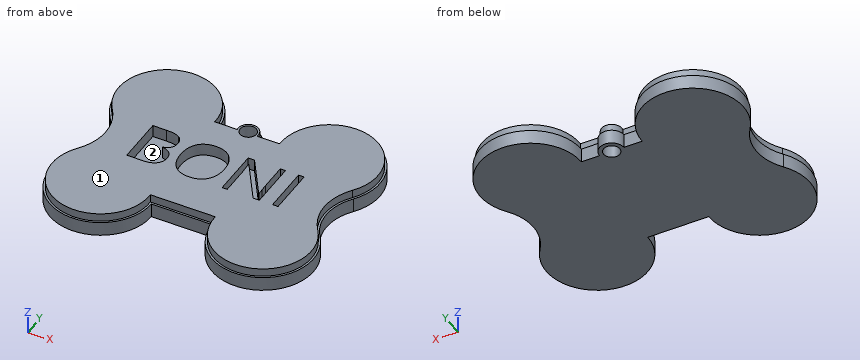
```python
from build123d import *

# Parameters (mm, degrees)
F0_R     = 2
F1_DEPTH = 3.5
F2_R     = 2
F3_DEPTH = 1
F4_W     = 1.3676754668
F4_H     = 11.7681905988
F4_R     = 2
F5_DEPTH = 3


with BuildPart() as f1:
    # F0 (on Top) → F1 (new body)
    with BuildSketch(Plane.XY):
        with BuildLine():
            Line((27, 30), (22.5, 30))
            ThreePointArc((22.5, 30), (6.0471529248, 41.8585412256), (0, 22.5))
            ThreePointArc((0, 22.5), (2.5, 15), (0, 7.5))
            ThreePointArc((0, 7.5), (6.0471529248, -11.8585412256), (22.5, 0))
            Line((22.5, 0), (37.5, 0))
            ThreePointArc((37.5, 0), (53.9528470752, -11.8585412256), (60, 7.5))
            ThreePointArc((60, 7.5), (57.5, 15), (60, 22.5))
            ThreePointArc((60, 22.5), (53.9528470752, 41.8585412256), (37.5, 30))
            Line((37.5, 30), (33, 30))
            ThreePointArc((33, 30), (30, 33), (27, 30))
        make_face()
        with Locations((30, 30)):
            Circle(F0_R, mode=Mode.SUBTRACT)
    extrude(amount=F1_DEPTH)

    # F2 (on face) → F3 (cut)
    with BuildSketch(Plane.XY.offset(3.5)):
        with BuildLine():
            Line((21.9895788083, 0.5), (38.0104211917, 0.5))
            ThreePointArc((38.0104211917, 0.5), (53.5566869022, -11.4608018166), (59.6, 7.2))
            ThreePointArc((59.6, 7.2), (57, 15), (59.6, 22.8))
            ThreePointArc((59.6, 22.8), (53.5566869022, 41.4608018166), (38.0104211917, 29.5))
            Line((38.0104211917, 29.5), (32.4494897428, 29.5))
            ThreePointArc((32.4494897428, 29.5), (30, 32.5), (27.5505102572, 29.5))
            Line((27.5505102572, 29.5), (21.9895788083, 29.5))
            ThreePointArc((21.9895788083, 29.5), (6.4433130978, 41.4608018166), (0.4, 22.8))
            ThreePointArc((0.4, 22.8), (3, 15), (0.4, 7.2))
            ThreePointArc((0.4, 7.2), (6.4433130978, -11.4608018166), (21.9895788083, 0.5))
        make_face()
        with Locations((30, 30)):
            Circle(F2_R, mode=Mode.SUBTRACT)
    extrude(amount=-F3_DEPTH, mode=Mode.SUBTRACT)

    # F4 (on face) → F5 (join)
    with BuildSketch(Plane.XY.offset(2.5)):
        with BuildLine():
            ThreePointArc((0.4, 7.2), (6.4433130978, -11.4608018166), (21.9895788083, 0.5))
            Line((21.9895788083, 0.5), (38.0104211917, 0.5))
            ThreePointArc((38.0104211917, 0.5), (53.5566869022, -11.4608018166), (59.6, 7.2))
            ThreePointArc((59.6, 7.2), (57, 15), (59.6, 22.8))
            ThreePointArc((59.6, 22.8), (53.5566869022, 41.4608018166), (38.0104211917, 29.5))
            Line((38.0104211917, 29.5), (32.4494897428, 29.5))
            ThreePointArc((32.4494897428, 29.5), (30, 32.5), (27.5505102572, 29.5))
            Line((27.5505102572, 29.5), (21.9895788083, 29.5))
            ThreePointArc((21.9895788083, 29.5), (6.4433130978, 41.4608018166), (0.4, 22.8))
            ThreePointArc((0.4, 22.8), (3, 15), (0.4, 7.2))
        make_face()
        with BuildLine():
            Line((10.8878203307, 10.1561439622), (10.8878203307, 21.924334561))
            Line((10.8878203307, 21.924334561), (14.2129974073, 21.924334561))
            add(Edge.make_bspline(
                [(14.2129974073, 21.924334561), (16.554272359, 21.924334561), (17.6012781542, 21.2237550375)],
                knots=[0, 0, 0, 1, 1, 1], degree=2))
            add(Edge.make_bspline(
                [(17.6012781542, 21.2237550375), (18.6482839495, 20.523175514), (18.6482839495, 19.0112630864)],
                knots=[0, 0, 0, 1, 1, 1], degree=2))
            add(Edge.make_bspline(
                [(18.6482839495, 19.0112630864), (18.6482839495, 17.9629694612), (18.0648969566, 17.2829952178)],
                knots=[0, 0, 0, 1, 1, 1], degree=2))
            add(Edge.make_bspline(
                [(18.0648969566, 17.2829952178), (17.4815099636, 16.6030209744), (16.361097858, 16.4021194934)],
                knots=[0, 0, 0, 1, 1, 1], degree=2))
            Line((16.361097858, 16.4021194934), (16.361097858, 16.322274033))
            add(Edge.make_bspline(
                [(16.361097858, 16.322274033), (19.0423599314, 15.8638065507), (19.0423599314, 13.5045019789)],
                knots=[0, 0, 0, 1, 1, 1], degree=2))
            add(Edge.make_bspline(
                [(19.0423599314, 13.5045019789), (19.0423599314, 11.928198051), (17.9760366861, 11.0421710066)],
                knots=[0, 0, 0, 1, 1, 1], degree=2))
            add(Edge.make_bspline(
                [(17.9760366861, 11.0421710066), (16.9097134408, 10.1561439622), (14.9934223912, 10.1561439622)],
                knots=[0, 0, 0, 1, 1, 1], degree=2))
            Line((14.9934223912, 10.1561439622), (10.8878203307, 10.1561439622))
        make_face(mode=Mode.SUBTRACT)
        with BuildLine():
            add(Edge.make_bspline(
                [(30.359810028, 20.4999945739), (31.7841500152, 18.8902070658), (31.7841500152, 16.0569810517)],
                knots=[0, 0, 0, 1, 1, 1], degree=2))
            add(Edge.make_bspline(
                [(31.7841500152, 16.0569810517), (31.7841500152, 13.2314820175), (30.354658708, 11.6126796994)],
                knots=[0, 0, 0, 1, 1, 1], degree=2))
            add(Edge.make_bspline(
                [(30.354658708, 11.6126796994), (28.9251674009, 9.9938773813), (26.3829909681, 9.9938773813)],
                knots=[0, 0, 0, 1, 1, 1], degree=2))
            add(Edge.make_bspline(
                [(26.3829909681, 9.9938773813), (23.7841500152, 9.9938773813), (22.3714004981, 11.5843474393)],
                knots=[0, 0, 0, 1, 1, 1], degree=2))
            add(Edge.make_bspline(
                [(22.3714004981, 11.5843474393), (20.958650981, 13.1748174973), (20.958650981, 16.0724350117)],
                knots=[0, 0, 0, 1, 1, 1], degree=2))
            add(Edge.make_bspline(
                [(20.958650981, 16.0724350117), (20.958650981, 18.9468715861), (22.3752639881, 20.528326834)],
                knots=[0, 0, 0, 1, 1, 1], degree=2))
            add(Edge.make_bspline(
                [(22.3752639881, 20.528326834), (23.7918769952, 22.1097820819), (26.3984449282, 22.1097820819)],
                knots=[0, 0, 0, 1, 1, 1], degree=2))
            add(Edge.make_bspline(
                [(26.3984449282, 22.1097820819), (28.9354700409, 22.1097820819), (30.359810028, 20.4999945739)],
                knots=[0, 0, 0, 1, 1, 1], degree=2))
        make_face(mode=Mode.SUBTRACT)
        with BuildLine():
            Line((43.5987024942, 21.924334561), (43.5987024942, 10.1561439622))
            Line((43.5987024942, 10.1561439622), (42.0378525264, 10.1561439622))
            Line((42.0378525264, 10.1561439622), (35.6064294743, 20.0312244515))
            Line((35.6064294743, 20.0312244515), (35.5420379739, 20.0312244515))
            add(Edge.make_bspline(
                [(35.5420379739, 20.0312244515), (35.6708209746, 18.2926539428), (35.6708209746, 16.8451330156)],
                knots=[0, 0, 0, 1, 1, 1], degree=2))
            Line((35.6708209746, 16.8451330156), (35.6708209746, 10.1561439622))
            Line((35.6708209746, 10.1561439622), (34.4061719083, 10.1561439622))
            Line((34.4061719083, 10.1561439622), (34.4061719083, 21.924334561))
            Line((34.4061719083, 21.924334561), (35.951567916, 21.924334561))
            Line((35.951567916, 21.924334561), (42.3675370081, 12.0878889718))
            Line((42.3675370081, 12.0878889718), (42.4319285084, 12.0878889718))
            add(Edge.make_bspline(
                [(42.4319285084, 12.0878889718), (42.4164745483, 12.3042444129), (42.359810028, 13.4838966988)],
                knots=[0, 0, 0, 1, 1, 1], degree=2))
            add(Edge.make_bspline(
                [(42.359810028, 13.4838966988), (42.3031455078, 14.6635489847), (42.3185994678, 15.1709540072)],
                knots=[0, 0, 0, 1, 1, 1], degree=2))
            Line((42.3185994678, 15.1709540072), (42.3185994678, 21.924334561))
            Line((42.3185994678, 21.924334561), (43.5987024942, 21.924334561))
        make_face(mode=Mode.SUBTRACT)
        with Locations((47.5175692038, 16.0402392616)):
            Rectangle(F4_W, F4_H, mode=Mode.SUBTRACT)
        with Locations((30, 30)):
            Circle(F4_R, mode=Mode.SUBTRACT)
    extrude(amount=F5_DEPTH)


solid = f1.part
```
CAD build for the part. Positions are in the model's coordinates, mm. Face numbers are marked on the shaded views. Coordinates: 2 decimals unless noted, no trailing zeros. Order: outer loops, then holes, each group sorted by start corner. A loop starts at its lowest first (then second) coordinate and runs counter-clockwise, first axis right, second up.
(1) Saw through at C-C, the plane x = 53.5. Write the cut outline in (y, z), and give its area (3 significant figures).
Solution:
outline: (-12, 0) - (42, 0) - (42, 3.5) - (41.48, 3.5) - (41.48, 5.5) - (-11.48, 5.5) - (-11.48, 3.5) - (-12, 3.5) - close
area: 295 mm2
(2) Pin check, flat tips, straight feed: pin 1 Ø1.6 at (x, z) = (24, 4.5) entering from +Y; pin 2 Ø0.9 at (y, z) = (13.5, 4.5) entering from +X; pin 3 Ø1 at (x, z) = (43, 4.5) entering from -Y; pin 4 Ø12 at (x, y) = (34, 5.5) entering from -Z. Stop position of each tip, or through.
Solution:
pin 1: stops at y = 29.5
pin 2: stops at x = 57.15
pin 3: stops at y = -10.09
pin 4: stops at z = 0
(3) Drill centre lines: L1, parallel to Y at x = 30, z = 1.45; L2, parallel to Y at x = 24, z = 1.55; L3, parallel to Y at x = 30, z = 4.15. Where is each one in solid material? Low to high.
Solution:
L1: y = 0 to 28, 32 to 33
L2: y = 0 to 30
L3: y = 0.5 to 11.25, 20.86 to 28, 32 to 32.5
(4) Mould opens along X. For the marked faces 1 and 2 say: released by +X, released by -X, zero draft, split by the parting line, or undercut.
Solution:
face 1: zero draft
face 2: undercut
(5) Saw through at A-A, the plane z = 0.85. Write the cut outline in (x, y), and give its area (3 significant figures).
Solution:
outline: (0, 7.5) arc R12.5 ccw (long way) to (22.5, 0) - (37.5, 0) arc R12.5 ccw (long way) to (60, 7.5) arc R12.5 cw to (60, 22.5) arc R12.5 ccw (long way) to (37.5, 30) - (33, 30) arc R3 ccw to (27, 30) - (22.5, 30) arc R12.5 ccw (long way) to (0, 22.5) arc R12.5 cw to start; hole circle Ø4 at (30, 30)
area: 2,780 mm2
(6) Saw through at B-B, the plane y = 26. Write the cut outline in (x, z), and give its area (3 significant figures).
Solution:
outline: (-1.84, 0) - (61.84, 0) - (61.84, 3.5) - (61.31, 3.5) - (61.31, 5.5) - (-1.31, 5.5) - (-1.31, 3.5) - (-1.84, 3.5) - close
area: 348 mm2
